Verification items for the finished model (mm, model axes). A direction names the side the tool comes from. Give positions to 0.01 mm unless a question says otherwise; leave off trailing zeros. Order: outer loops, then holes, each group sorted by start corner. A loop starts at its lowest first (then second) coordinate and runs counter-clockwise, first axis right, second up. Notation, with made-up numbers: (6, 65.5) - (62, 65.5) arc R32 cw to (62, 101.5) - close; hole circle Ø5 at (78.5, 69.25). An arc over 180 degrees is marked (long way). Answer as a JSON object with one key per item and string values. Group by question number.
(1) Mould release check, pull along X, two halves, no side actions. Record for faces 1 (the face through (5, -2, 0)), 2 (the face through (-25, 2, 0)), 3 (the face through (-15, 15, 0)), 4 (the face through (20, 12, 0)): +X half, -X half, draft (parallel to the pull), parting line (faces both ways), or undercut.
(2) Section check A-A (y = 13.5). Record the boundary of the cut face in (x, z).
(3) Section check D-D (x = -8.5). Record the boundary of the cut face in (y, z).
(4) Thickness scan on line 1 (X direction, y = 13, z = -3.5); line 2 (X direction, y = -2, z = -0.75); line 3 (Z direction, x = 10.5, y = -2). Record the ranges inside material, lowest first.
(5) Depth check by flat-ended pin: pin 1 Ø1.5 at (y, z) = (13, -2) entering from +X; pin 2 Ø5.5 at (x, y) = (14, 13.5) entering from +Z; pin 3 Ø8 at (x, z) = (-14.5, 0) entering from -Y. Enter the tip coordinate at first touch or a pass-through.
(6) Section check B-B (z = -3.75). Record the boundary of the cut face in (x, y).
(7) Access from +Z, -Z, +X, -X, +Y, -Y to the whole of each face (thin tool, end or side, straight path). Record for faces 5 (the face through (-20, 12, 0)), 6 (the face through (15, 0, 0)), 7 (the face through (-10, 12, 0)), 8 (the face through (-15, 12, -5)), 9 (the face through (0, 12, 5)).
(8) Section check C-C (y = -3.5). Record the boundary of the cut face in (x, z).
```python
from build123d import *

# Parameters (mm, degrees)
F0_W     = 50
F0_H     = 20
F0_W_2   = 10
F0_H_2   = 10
F1_DEPTH = 5
F2_W     = 50
F2_H     = 20
F3_DEPTH = 10
F4_W     = 10
F4_H     = 10
F5_DEPTH = 5


with BuildPart() as f1:
    # F0 (on Front) → F1 (new body)
    with BuildSketch(Plane.XZ):
        Rectangle(F0_W, F0_H)
        with Locations((-15, 0)):
            Rectangle(F0_W_2, F0_H_2, mode=Mode.SUBTRACT)
        Rectangle(F0_W_2, F0_H_2, mode=Mode.SUBTRACT)
        with Locations((15, 0)):
            Rectangle(F0_W_2, F0_H_2, mode=Mode.SUBTRACT)
    extrude(amount=F1_DEPTH)

    # F2 (on face) → F3 (join)
    with BuildSketch(Plane(origin=(0, 0, 0), x_dir=(-1, 0, 0), z_dir=(0, 1, 0))):
        Rectangle(F2_W, F2_H)
    extrude(amount=F3_DEPTH)

    # F4 (on face) → F5 (join)
    with BuildSketch(Plane(origin=(0, 10, 0), x_dir=(-1, 0, 0), z_dir=(0, 1, 0))):
        Rectangle(F4_W, F4_H)
        with Locations((-15, 0)):
            Rectangle(F4_W, F4_H)
        with Locations((15, 0)):
            Rectangle(F4_W, F4_H)
    extrude(amount=F5_DEPTH)


solid = f1.part
```
Solutions:
{
 "1": {"face 1": "undercut", "face 2": "-X half", "face 3": "draft", "face 4": "+X half"},
 "2": {"outline": "(-20, -5) - (-10, -5) - (-10, 5) - (-20, 5) - close; (-5, -5) - (5, -5) - (5, 5) - (-5, 5) - close; (10, -5) - (20, -5) - (20, 5) - (10, 5) - close"},
 "3": {"outline": "(-5, -10) - (10, -10) - (10, 10) - (-5, 10) - close"},
 "4": {"line 1": "x = -20 to -10, -5 to 5, 10 to 20", "line 2": "x = -25 to -20, -10 to -5, 5 to 10, 20 to 25", "line 3": "z = -10 to -5, 5 to 10"},
 "5": {"pin 1": "stops at x = 20", "pin 2": "stops at z = 5", "pin 3": "stops at y = 0"},
 "6": {"outline": "(-25, -5) - (-20, -5) - (-20, 0) - (-10, 0) - (-10, -5) - (-5, -5) - (-5, 0) - (5, 0) - (5, -5) - (10, -5) - (10, 0) - (20, 0) - (20, -5) - (25, -5) - (25, 10) - (20, 10) - (20, 15) - (10, 15) - (10, 10) - (5, 10) - (5, 15) - (-5, 15) - (-5, 10) - (-10, 10) - (-10, 15) - (-20, 15) - (-20, 10) - (-25, 10) - close"},
 "7": {"face 5": "+Z, -Z, -X, +Y", "face 6": "-Y", "face 7": "+Z, -Z, +Y", "face 8": "-Z, +X, -X, +Y", "face 9": "+Z, +X, -X, +Y"},
 "8": {"outline": "(-25, -10) - (25, -10) - (25, 10) - (-25, 10) - close; hole (-20, -5) - (-10, -5) - (-10, 5) - (-20, 5) - close; hole (-5, -5) - (5, -5) - (5, 5) - (-5, 5) - close; hole (10, -5) - (20, -5) - (20, 5) - (10, 5) - close"}
}
